Here's how the part is built. I have some questions about the finished solid (model axes, mm). Face numbers are marked on the shaded views. A direction names the side the tool comes from. Coordinates: 2 decimals unless noted, no trailing zeros. Loops run counter-clockwise (first coordinate to the right, second up) from the corner with the lowest first, then second, coordinate; pieces in that order, holes last. Notation, with made-up numbers: M 18,61.5 L 60,61.5 A15 cw 60,83.5 Z; hole C 35.25,-14 d6. An arc over 180 degrees is marked long. Use CSV: the item, a comma, the result in double quotes. Start each with the question number.
Q1. Please list where these lines run through material, in increasing order: probe 1 along Z at (x, y) = (5.5, -102); probe 2 along Z at (x, y) = (-4.25, -105); probe 3 along Y at (x, z) = (0, 36.75). Write a range as [from, to].
Q2. If we section it at A-A (x = 0): Please give me the cut outline in (y, z), and give its area (3 significant figures).
Q3. For pin 1 Ø1.5 at (x, z) = (-0.5, 33.5) entering from -Y; pin 2 Ø5 at (x, y) = (-1, -103.5) entering from -Z; pin 3 Ø3.5 at (x, y) = (0, -103) entering from -Z; pin 4 Ø4 at (x, z) = (5, 40.5) entering from +Y, each with a flat end and sliding along its axis, tell me the tip position at first contact or that it passes through.
Q4. If we section it at D-D (x = -3.25): Please give me the cut outline in (y, z), and give its area (3 significant figures).
Q5. If we section it at C-C (y = -107.5): Please give me the cut outline in (x, z), and give its area (3 significant figures).
Q6. Which directions (+Z, -Z, +X, -X, +Y, -Y) give clear straight access to the entire face, cutting with the end or side of a thin tool? Please do the marked faces 1, 2, 3, 4 and 5.
Q7. If we section it at B-B (z = 47.75): Please give me the cut outline in (x, y).
Q8. If we mould it in two halves opening along Y, with no side actions, what happens to the marked faces 6, 7 and 8? For each: +Y half, -Y half, draft (parallel to the pull), parting line (faces both ways), or undercut.
from build123d import *

# Parameters (mm, degrees)
SKETCH151_R             = 2
PAD064_DEPTH            = 4
SKETCH152_R             = 5
SKETCH152_R_2           = 2
PAD065_DEPTH            = 4
SKETCH153_R             = 4
SKETCH153_R_2           = 2
PAD066_DEPTH            = 9
SKETCH157_R             = 2.25
POCKET066_DEPTH         = 10
SKETCH164_R             = 5
POCKET067_DEPTH         = 3
BODY018_PLACEMENT_ANGLE = 90


with BuildPart() as part:
    # Sketch151 → Pad064 (new body)
    with BuildSketch(Plane.XZ):
        Polygon((7, 0), (3.5, 6.062178), (-3.5, 6.062178), (-7, 0), (-3.5, -6.062178), (3.5, -6.062178), align=None)
        Circle(SKETCH151_R, mode=Mode.SUBTRACT)
    extrude(amount=PAD064_DEPTH)

    # Sketch152 (on Face9 of Pad064) → Pad065 (join)
    with BuildSketch(Plane.XZ.offset(4)):
        Circle(SKETCH152_R)
        Circle(SKETCH152_R_2, mode=Mode.SUBTRACT)
    extrude(amount=PAD065_DEPTH)

    # Sketch153 (on Face12 of Pad065) → Pad066 (join)
    with BuildSketch(Plane.XZ.offset(8)):
        Circle(SKETCH153_R)
        Circle(SKETCH153_R_2, mode=Mode.SUBTRACT)
    extrude(amount=PAD066_DEPTH)

    # Sketch157 (on Face15 of Pad066) → Pocket066 (cut)
    with BuildSketch(Plane.XZ.offset(17)):
        Circle(SKETCH157_R)
    extrude(amount=-POCKET066_DEPTH, mode=Mode.SUBTRACT)

    # Sketch164 (on Face16 of Pocket066) → Pocket067 (cut)
    with BuildSketch(Plane.XZ.offset(17)):
        Circle(SKETCH164_R)
        Polygon((4, 0), (2, 3.464102), (-2, 3.464102), (-4, 0), (-2, -3.464102), (2, -3.464102), align=None, mode=Mode.SUBTRACT)
    extrude(amount=-POCKET067_DEPTH, mode=Mode.SUBTRACT)


with BuildPart() as part_1:
    # Body018 placement: moved
    add(part.part.moved(Location((0, -103, 49))).rotate(Axis((0, -103, 49), (1, 0, 0)), BODY018_PLACEMENT_ANGLE))


solid = part_1.part
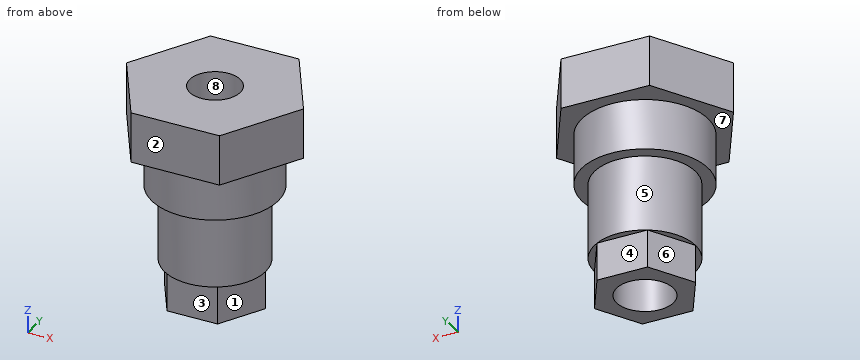
Results below:
1,probe 1,"[45, 49]"
1,probe 2,"[41, 49]"
1,probe 3,"[-107, -105.25], [-100.75, -99]"
2,outline,"M -109.06,45 L -108,45 L -108,41 L -107,41 L -107,35 L -106.46,35 L -106.46,32 L -105.25,32 L -105.25,42 L -105,42 L -105,49 L -109.06,49 Z; M -101,42 L -100.75,42 L -100.75,32 L -99.54,32 L -99.54,35 L -99,35 L -99,41 L -98,41 L -98,45 L -96.94,45 L -96.94,49 L -101,49 Z"
2,area,"84.3 mm^2"
3,pin 1,"y = -106.46"
3,pin 2,"z = 32"
3,pin 3,"through"
3,pin 4,"y = -99.05"
4,outline,"M -109.06,45 L -106.8,45 L -106.8,41 L -105.33,41 L -105.33,35 L -104.3,35 L -104.3,32 L -101.7,32 L -101.7,35 L -100.67,35 L -100.67,41 L -99.2,41 L -99.2,45 L -96.94,45 L -96.94,49 L -109.06,49 Z"
4,area,"115 mm^2"
5,outline,"M -4.4,45 L -2.18,45 L -2.18,41 L 2.18,41 L 2.18,45 L 4.4,45 L 4.4,49 L -4.4,49 Z"
5,area,"52.7 mm^2"
6,face 1,"-Z, +X, -Y"
6,face 2,"+Z, -Z, +X, -X, -Y"
6,face 3,"-Z, +X, -X, -Y"
6,face 4,"-Z, +X, -X, +Y"
6,face 5,"-Z"
7,outline,"M -7,-103 L -3.5,-109.06 L 3.5,-109.06 L 7,-103 L 3.5,-96.94 L -3.5,-96.94 Z; hole C 0,-103 d4"
8,face 6,"+Y half"
8,face 7,"draft"
8,face 8,"undercut"
